```python
from build123d import *

# Parameters (mm, degrees)
SKETCH_1_W                = 27
SKETCH_1_H                = 15
EXTRUDE_1_DEPTH           = 8
CUT_EXTRUDE_8_DEPTH       = 41.5
SKETCH_5_W                = 4
SKETCH_5_H                = 15
EXTRUDE_3_DEPTH           = 24
SKETCH_7_W                = 5
SKETCH_7_H                = 6.5
CUT_EXTRUDE_5_DEPTH       = 1.5
SKETCH_10_R               = 1.5
CUT_EXTRUDE_6_DEPTH       = 21.5
SKETCH_12_W               = 5
SKETCH_12_H               = 10
CUT_EXTRUDE_7_DEPTH       = 21.5
SKETCH_14_W               = 4
SKETCH_14_H               = 2
CUT_EXTRUDE_9_DEPTH       = 21.5
SKETCH_15_R               = 1.5
CUT_EXTRUDE_10_DEPTH      = 21.5
EXTRUDE_6_DEPTH           = 4
CUT_EXTRUDE_13_DEPTH      = 1.5
CUT_EXTRUDE_13_DEPTH_BACK = 12
SKETCH_17_R               = 3
CUT_EXTRUDE_15_DEPTH      = 1
CUT_EXTRUDE_15_DEPTH_BACK = 2.5
SKETCH_19_R               = 3
CUT_EXTRUDE_16_DEPTH      = 54
SKETCH_23_W               = 9
SKETCH_23_H               = 12
CUT_EXTRUDE_17_DEPTH      = 1
FILLET_2_R                = 2
FILLET_3_R                = 2
FILLET_4_R                = 5
CHAMFER_1_SIZE            = 1.5
FILLET_5_R                = 2
FILLET_8_R                = 1


with BuildPart() as part:
    # 草图1 → 凸台-拉伸1 (new body)
    with BuildSketch(Plane(origin=(0, 0, 0), x_dir=(1, 0, 0), z_dir=(0, 1, 0))):
        Rectangle(SKETCH_1_W, SKETCH_1_H)
    extrude(amount=EXTRUDE_1_DEPTH)

    # 草图13 → 切除-拉伸8 (cut)
    with BuildSketch(Plane(origin=(13.5, 0, 0), x_dir=(0, 0, -1), z_dir=(1, 0, 0))):
        Polygon((-7.5, 4), (7.5, 0), (-7.5, 0), align=None)
    extrude(amount=-CUT_EXTRUDE_8_DEPTH, mode=Mode.SUBTRACT)

    # 草图5 → 凸台-拉伸3 (add)
    with BuildSketch(Plane(origin=(0, 8, 0), x_dir=(1, 0, 0), z_dir=(0, 1, 0))):
        with Locations((11.5, 0)):
            Rectangle(SKETCH_5_W, SKETCH_5_H)
    extrude(amount=EXTRUDE_3_DEPTH)

    # 草图7 → 切除-拉伸5 (cut)
    with BuildSketch(Plane(origin=(0, 8, 0), x_dir=(1, 0, 0), z_dir=(0, 1, 0))):
        with Locations((1.5, 0.25)):
            Rectangle(SKETCH_7_W, SKETCH_7_H)
    extrude(amount=-CUT_EXTRUDE_5_DEPTH, mode=Mode.SUBTRACT)

    # 草图10 → 切除-拉伸6 (cut)
    with BuildSketch(Plane.ZY.offset(-13.5)):
        with Locations(Location((4.5, 14, 0), (0, 0, 180))):
            Circle(SKETCH_10_R)
        with Locations(Location((4.5, 26, 0), (0, 0, 180))):
            Circle(SKETCH_10_R)
    extrude(amount=CUT_EXTRUDE_6_DEPTH, mode=Mode.SUBTRACT)

    # 草图12 → 切除-拉伸7 (cut)
    with BuildSketch(Plane.ZY.offset(-9.5)):
        with Locations((-4, 20)):
            Rectangle(SKETCH_12_W, SKETCH_12_H)
    extrude(amount=-CUT_EXTRUDE_7_DEPTH, mode=Mode.SUBTRACT)

    # 草图14 → 切除-拉伸9 (cut)
    with BuildSketch(Plane.XY.offset(7.5)):
        with Locations((11.5, 31)):
            Rectangle(SKETCH_14_W, SKETCH_14_H)
    extrude(amount=-CUT_EXTRUDE_9_DEPTH, mode=Mode.SUBTRACT)

    # 草图15 → 切除-拉伸10 (cut)
    with BuildSketch(Plane(origin=(0, 1.867219917, -0.497925311), x_dir=(1, 0, 0), z_dir=(0, -0.9662349396012463, 0.25766265056033233))):
        with Locations(Location((-4.971460236, 0.653668071, 0), (0, 0, 270))):
            Circle(SKETCH_15_R)
        with Locations(Location((2.5, 0, 0), (0, 0, 270))):
            Circle(SKETCH_15_R)
    extrude(amount=-CUT_EXTRUDE_10_DEPTH, mode=Mode.SUBTRACT)

    # 草图21 → 凸台-拉伸6 (add)
    with BuildSketch(Plane(origin=(0, 0, -7.5), x_dir=(-1, 0, 0), z_dir=(0, 0, -1))):
        Polygon((-13.5, -1.987071707), (11.82839978, -1.987071707), (13.5, -1.987071707), (13.5, 8), (-9.5, 8), (-9.5, 30), (-13.5, 30), (-13.5, 8), align=None)
    extrude(amount=EXTRUDE_6_DEPTH)

    # 草图17 → 切除-拉伸13 (cut, two sides: drawn at the far end of the back side and taken through both)
    with BuildSketch(Plane(origin=(0, 6.698394615, -1.786238564), x_dir=(-1, 0, 0), z_dir=(0, -0.9662349396012463, 0.25766265056033233)).offset(-CUT_EXTRUDE_13_DEPTH_BACK)):
        with Locations(Location((-2.5, 0, 0), (0, 0, 240))):
            Circle(SKETCH_17_R)
    extrude(amount=CUT_EXTRUDE_13_DEPTH + CUT_EXTRUDE_13_DEPTH_BACK, mode=Mode.SUBTRACT)

    # 草图19 → 切除-拉伸15 (cut, two sides: drawn at the far end of the back side and taken through both)
    with BuildSketch(Plane(origin=(0, 6.698394615, -1.786238564), x_dir=(-1, 0, 0), z_dir=(0, -0.9662349396012463, 0.25766265056033233)).offset(-CUT_EXTRUDE_15_DEPTH_BACK)):
        with Locations(Location((4.971460236, -0.653668071, 0), (0, 0, 90))):
            Circle(SKETCH_19_R)
    extrude(amount=CUT_EXTRUDE_15_DEPTH + CUT_EXTRUDE_15_DEPTH_BACK, mode=Mode.SUBTRACT)

    # 草图22 → 切除-拉伸16 (cut)
    with BuildSketch(Plane(origin=(13.5, 0, 0), x_dir=(0, 0, -1), z_dir=(1, 0, 0))):
        Polygon((-7.5, 4), (7.5, 0), (11.5, -1.066666667), (11.5, -3.267506917), (3.736378374, -2.578943079), align=None)
    extrude(amount=-CUT_EXTRUDE_16_DEPTH, mode=Mode.SUBTRACT)

    # 草图23 → 切除-拉伸17 (cut)
    with BuildSketch(Plane.ZY.offset(-13.5)):
        with Locations((-4, 20)):
            Rectangle(SKETCH_23_W, SKETCH_23_H)
    extrude(amount=CUT_EXTRUDE_17_DEPTH, mode=Mode.SUBTRACT)

    # 圆角2
    fillet_2_edges = [part.edges().sort_by_distance(p)[0] for p in [
        (9.5, 8, -2),
    ]]
    fillet(fillet_2_edges, radius=FILLET_2_R)

    # 圆角3
    fillet_3_edges = [part.edges().sort_by_distance(p)[0] for p in [
        (13.5, 30, -2),
    ]]
    fillet(fillet_3_edges, radius=FILLET_3_R)

    # 圆角4
    fillet_4_edges = [part.edges().sort_by_distance(p)[0] for p in [
        (13.5, 1.466666667, -2),
    ]]
    fillet(fillet_4_edges, radius=FILLET_4_R)

    # 倒角1
    # the kernel refuses this chamfer: 1.5 mm, written as the material it takes off along each edge
    with BuildSketch(Plane(origin=(2.5, 5.249042206, -1.399744588), x_dir=(0, -0.2576626505603323, -0.9662349396012463), z_dir=(-1, 0, 0))) as chamfer_1_piece_1_section:
        Polygon((1.5, CHAMFER_1_SIZE), (1.5 + CHAMFER_1_SIZE, 0), (1.5, 0), align=None)
    chamfer_1_piece_1 = revolve(axis=Axis((2.5, 5.249042206, -1.399744588), (0, -0.9662349396012463, 0.25766265056033233)), mode=Mode.PRIVATE)
    chamfer_1_piece_1 = chamfer_1_piece_1 & Plane(origin=(2.5, 4.520895406, -1.205572108), x_dir=(0.5000000000000004, 0.22314240099168048, 0.8367840037188018), z_dir=(0, -0.9662349396012463, 0.25766265056033233)) * Cylinder(3, 12, mode=Mode.PRIVATE)
    add(chamfer_1_piece_1, mode=Mode.SUBTRACT)
    with BuildSketch(Plane(origin=(-4.971460236, 5.900585523, -0.896978985), x_dir=(0, -0.25766265056033244, -0.9662349396012462), z_dir=(-1, 0, 0))) as chamfer_1_piece_2_section:
        Polygon((1.5, CHAMFER_1_SIZE), (1.5 + CHAMFER_1_SIZE, 0), (1.5, 0), align=None)
    chamfer_1_piece_2 = revolve(axis=Axis((-4.971460236, 5.900585523, -0.896978985), (0, -0.9662349396012463, 0.25766265056033233)), mode=Mode.PRIVATE)
    chamfer_1_piece_2 = chamfer_1_piece_2 & Plane(origin=(-4.971460236, 5.172438723, -0.702806505), x_dir=(0, -0.25766265056033233, -0.9662349396012463), z_dir=(0, 0.9662349396012463, -0.25766265056033233)) * Cylinder(3, 13, mode=Mode.PRIVATE)
    add(chamfer_1_piece_2, mode=Mode.SUBTRACT)
    with BuildSketch(Plane(origin=(13.5, 14, 4.5), x_dir=(0, 0, -1), z_dir=(0, 1, 0))) as chamfer_1_piece_3:
        Polygon((1.5 + CHAMFER_1_SIZE, 0), (1.5, CHAMFER_1_SIZE), (1.5, 0), align=None)
    revolve(axis=Axis((13.5, 14, 4.5), (-1, 0, 0)), mode=Mode.SUBTRACT)
    with BuildSketch(Plane(origin=(13.5, 26, 4.5), x_dir=(0, 0, -1), z_dir=(0, 1, 0))) as chamfer_1_piece_4:
        Polygon((1.5 + CHAMFER_1_SIZE, 0), (1.5, CHAMFER_1_SIZE), (1.5, 0), align=None)
    revolve(axis=Axis((13.5, 26, 4.5), (-1, 0, 0)), mode=Mode.SUBTRACT)

    # 圆角5
    # the kernel refuses this fillet: 2 mm, written as the material it takes off along each edge
    with BuildSketch(Plane(origin=(-11.5, 1.536556626, -9.5), x_dir=(0, 0, -1), z_dir=(-1, 0, 0))) as fillet_5_piece_1_section:
        Polygon((0, 0), (FILLET_5_R * 1.02, 0), (FILLET_5_R * 1.02, FILLET_5_R * 1.32764387935), (-FILLET_5_R * 0.262815903572, FILLET_5_R * 0.985559638393), align=None)
    fillet_5_piece_1 = extrude(amount=FILLET_5_R * 1.02, mode=Mode.PRIVATE)
    fillet_5_piece_1 = fillet_5_piece_1 - Plane(origin=(-11.5, 1.536556626, -9.5), x_dir=(0, 0.7929888557099438, 0.6092361403592483), z_dir=(-1, 0, 0)) * Sphere(FILLET_5_R, mode=Mode.PRIVATE)
    add(fillet_5_piece_1, mode=Mode.SUBTRACT)
    with BuildSketch(Plane(origin=(-13.5, -0.395913253, -8.984674699), x_dir=(1, 0, 0), z_dir=(0, 0.2576626505603323, 0.9662349396012463))) as fillet_5_piece_2:
        with BuildLine():
            CenterArc((FILLET_5_R, FILLET_5_R), FILLET_5_R, 180, 90)
            Line((0, FILLET_5_R), (0, 0))
            Line((0, 0), (FILLET_5_R, 0))
        make_face()
    extrude(amount=22.060731322, mode=Mode.SUBTRACT)
    with BuildSketch(Plane(origin=(12.341391565, 4, 7.5), x_dir=(0, 1, 0), z_dir=(-1, 0, 0))) as fillet_5_piece_3:
        with BuildLine():
            CenterArc((FILLET_5_R * 0.768278313084, FILLET_5_R), FILLET_5_R, 194.931417178, 75.068582822)
            Line((-FILLET_5_R * 0.197956626517, FILLET_5_R * 0.74233734944), (0, 0))
            Line((0, 0), (FILLET_5_R * 0.768278313084, 0))
        make_face()
    extrude(amount=29.682783131, mode=Mode.SUBTRACT)
    with BuildSketch(Plane(origin=(15.008058232, -1.066666667, -11.5), x_dir=(0, 0.25766265056033255, 0.9662349396012463), z_dir=(-1, 0, 0))) as fillet_5_piece_4:
        with BuildLine():
            CenterArc((FILLET_5_R * 1.30161164642, FILLET_5_R), FILLET_5_R, 165.068582822, 104.931417178)
            Line((FILLET_5_R * 0.335376706816, FILLET_5_R * 1.25766265056), (0, 0))
            Line((0, 0), (FILLET_5_R * 1.30161164642, 0))
        make_face()
    extrude(amount=26.508058232, mode=Mode.SUBTRACT)
    with BuildSketch(Plane(origin=(-13.5, 1.536556626, -11.5), x_dir=(0, 0, 1), z_dir=(0, 1, 0))) as fillet_5_piece_5:
        with BuildLine():
            CenterArc((FILLET_5_R, FILLET_5_R), FILLET_5_R, 180, 90)
            Line((0, FILLET_5_R), (0, 0))
            Line((0, 0), (FILLET_5_R, 0))
        make_face()
    extrude(amount=11.463443374, mode=Mode.SUBTRACT)

    # 圆角8
    fillet_8_edges = [part.edges().sort_by_distance(p)[0] for p in [
        (11, 25, -1.5),
        (11, 25, -6.5),
        (11, 15, -6.5),
        (11, 15, -1.5),
        (13, 14, 0.5),
        (13, 26, 0.5),
        (13, 26, -8.5),
        (13, 14, -8.5),
    ]]
    fillet(fillet_8_edges, radius=FILLET_8_R)


solid = part.part
```
Here's how the part is built. I have some questions about the finished solid (model axes, mm). A direction names the side the tool comes from. Coordinates: 2 decimals unless noted, no trailing zeros. Loops run counter-clockwise (first coordinate to the right, second up) from the corner with the lowest first, then second, coordinate; pieces in that order, holes last. Notation, with made-up numbers: M -34.75,49.25 L 22.25,49.25 A32 cw 22.25,77.25 Z; hole C -31.75,-33.75 d10. An arc over 180 degrees is marked long. One line per item, written item: value.
1. Imagine slicing it at A-A (y = 20). List the corners of the cut face in (x, z) for me.
Geometry says:
outline: M 9.5,-11.5 L 13.5,-11.5 L 13.5,-8.5 L 12.5,-8.5 L 12.5,-6.5 L 9.5,-6.5 Z; M 9.5,-1.5 L 12.5,-1.5 L 12.5,0.5 L 13.5,0.5 L 13.5,7.5 L 9.5,7.5 Z
2. Thinking about a two-plate mould opening in Y: for faces 1 (the flat face through (-1, 7, 0)), 2 (the flat face through (13, 20, -8.5)), 3 (the flat face through (0.9, 6.5, 1.1)), which applies, +Y half, -Y half, draft (parallel to the pull), parting line (faces both ways), or undercut?
Geometry says:
face 1: draft
face 2: undercut
face 3: +Y half
3. Please list where these lines run through material, in increasing order: probe 1 along Z at (x, y) = (10.1, 26); probe 2 along Y at (x, z) = (11.5, 4.5); probe 3 along Y at (x, z) = (11.25, 4.5).
Geometry says:
probe 1: z = -11.5 to 3, 6 to 7.5
probe 2: y = 4.23 to 12.5, 15.5 to 24.5, 27.5 to 30
probe 3: y = 4.05 to 12.5, 15.5 to 24.5, 27.5 to 30
4. On a 3-axis mill with a long thin cutter (end or side, diameter ignored), from which of +Z, -Z, +X, -X, +Y, -Y can I reach the whole of each face in a straight line? I mean faces 4 (the flat face through (13, 14, -4)), 5 (the flat face through (9.5, 20, 0)), 6 (the cylindrical face through (11.021, 15.301, -6.215)), 7 (the flat face through (10, 13, 7.5)), 8 (the flat face through (1, 7, 3)). Say none if no direction works.
Geometry says:
face 4: +X
face 5: +Z, -Z, -X, +Y
face 6: +X, -X
face 7: +Z, +X, -X, +Y, -Y
face 8: +Y
5. Will these pins go through, and if not, where does the flat tip stop? pin 1 Ø1.5 at (x, z) = (-0.5, -8.5) entering from +Y; pin 2 Ø2 at (x, z) = (-7.5, -3) entering from -Y; pin 3 Ø1.1 at (x, z) = (13, -4.5) entering from -Y; pin 4 Ø10 at (x, y) = (3.5, 23.5) entering from -Z.
Geometry says:
pin 1: stops at y = 8
pin 2: stops at y = 0.93
pin 3: stops at y = 2.79
pin 4: passes through
6. Imagine slicing it at B-B (x = -8.5). List the corners of the cut face in (y, z) for me.
Geometry says:
outline: M -0.4,-8.98 A2 ccw 1.54,-11.5 L 8,-11.5 L 8,7.5 L 5.54,7.5 A2 ccw 3.6,6.02 Z
7. Imagine slicing it at C-C (z = 4.5). State how many separate pieces and enclosed holes the cut face has, and give its area (3 significant figures).
Geometry says:
separate pieces: 3
enclosed holes: 0
area: 183 mm2
